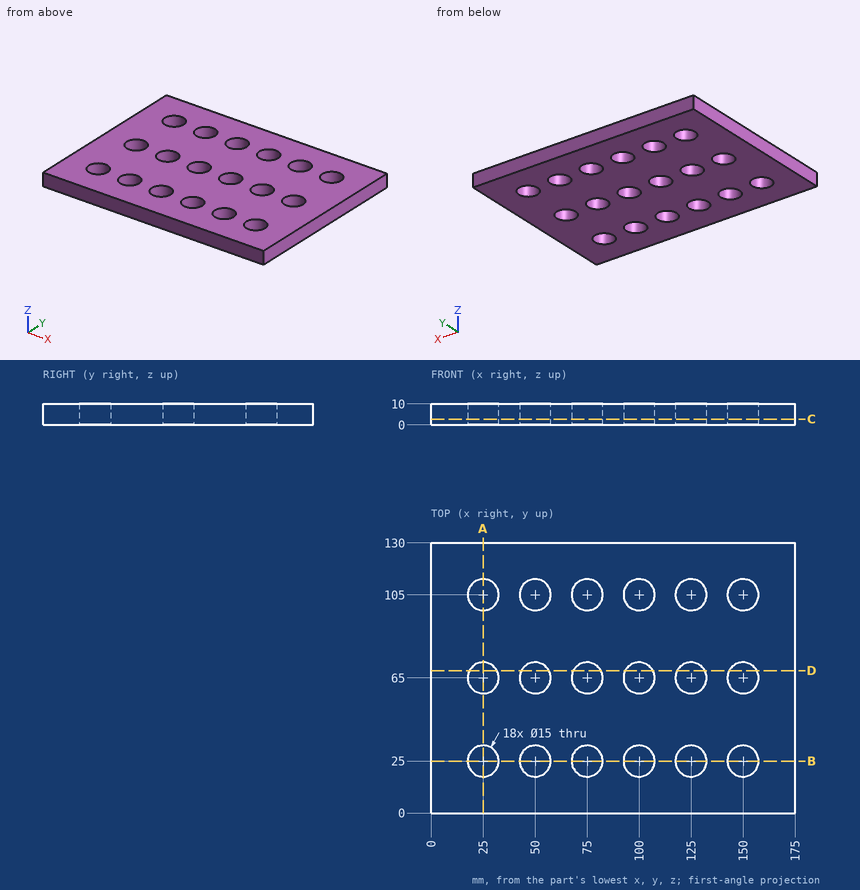
Could you check a few things on this drawing? It's one solid part, dimensions in mm from its lowest x, y, z. Coordinates: 2 decimals unless noted, no trailing zeros. Order: outer loops, then holes, each group sorted by start corner. A loop starts at its lowest first (then second) coordinate and runs counter-clockwise, first axis right, second up. Notation, with made-up numbers: (-22.75, 21) - (18.25, 21) arc R27 cw to (18.25, 52) - close; hole circle Ø6 at (38, -25). An arc over 180 degrees is marked (long way). One line per question, with ' | ' between items. Start each with the question number.
1. I'm going to push a flat-ended pin straight in: pin 1 Ø13.5 at (x, y) = (50, 65) entering from -Z. Where does the tip first touch, or does it pass through?
2. If we section it at B-B (y = 25): Write out the boundary of the cut face in (x, z).
3. If we section it at D-D (y = 68.5): Write out the boundary of the cut face in (x, z).
4. If we section it at C-C (z = 2.75): Give the number of separate pieces and of enclosed holes in the cut face, and give its area (3 significant figures).
5. If we section it at A-A (x = 25): Write out the boundary of the cut face in (y, z), and give its area (3 significant figures).
6. Please list where these lines run through material, in increasing order: line 1 along Y through (x, z) = (50, 3.5); line 2 along Y through (x, z) = (46.5, 6.5). Write a range as [from, to].
Model answer:
1) pin 1: passes through
2) outline: (0, 0) - (17.5, 0) - (17.5, 10) - (0, 10) - close; (32.5, 0) - (42.5, 0) - (42.5, 10) - (32.5, 10) - close; (57.5, 0) - (67.5, 0) - (67.5, 10) - (57.5, 10) - close; (82.5, 0) - (92.5, 0) - (92.5, 10) - (82.5, 10) - close; (107.5, 0) - (117.5, 0) - (117.5, 10) - (107.5, 10) - close; (132.5, 0) - (142.5, 0) - (142.5, 10) - (132.5, 10) - close; (157.5, 0) - (175, 0) - (175, 10) - (157.5, 10) - close
3) outline: (0, 0) - (18.37, 0) - (18.37, 10) - (0, 10) - close; (31.63, 0) - (43.37, 0) - (43.37, 10) - (31.63, 10) - close; (56.63, 0) - (68.37, 0) - (68.37, 10) - (56.63, 10) - close; (81.63, 0) - (93.37, 0) - (93.37, 10) - (81.63, 10) - close; (106.63, 0) - (118.37, 0) - (118.37, 10) - (106.63, 10) - close; (131.63, 0) - (143.37, 0) - (143.37, 10) - (131.63, 10) - close; (156.63, 0) - (175, 0) - (175, 10) - (156.63, 10) - close
4) separate pieces: 1 | enclosed holes: 18 | area: 19,600 mm²
5) outline: (0, 0) - (17.5, 0) - (17.5, 10) - (0, 10) - close; (32.5, 0) - (57.5, 0) - (57.5, 10) - (32.5, 10) - close; (72.5, 0) - (97.5, 0) - (97.5, 10) - (72.5, 10) - close; (112.5, 0) - (130, 0) - (130, 10) - (112.5, 10) - close | area: 850 mm²
6) line 1: y = [0, 17.5], [32.5, 57.5], [72.5, 97.5], [112.5, 130] | line 2: y = [0, 18.37], [31.63, 58.37], [71.63, 98.37], [111.63, 130]
